Check sheet for the modelled part. Datum: model origin and axes. Units: mm. A direction names the side the tool comes from. Give positions to 0.01 mm unless a question says otherwise; leave off trailing zeros. Loops run counter-clockwise (first coordinate to the right, second up) from the corner with the lowest first, then second, coordinate; pieces in that order, holes last. Notation, with made-up numbers: (70, -7.5) - (101, -7.5) arc R21 cw to (101, -2.5) - close; hole circle Ø3 at (-20, 8.25). An arc over 180 degrees is marked (long way). Use one line per item in the form item = value.
from build123d import *

# Parameters (mm, degrees)
F0_W     = 698.5
F0_H     = 787.4
F1_DEPTH = 6.35
F2_W     = 660.4
F2_H     = 19.05
F3_DEPTH = 228.6
F4_W     = 152.4
F4_H     = 76.2
F5_DEPTH = 25.4


with BuildPart() as f1:
    # F0 (on Front) → F1 (new body)
    with BuildSketch(Plane.XZ):
        with Locations((349.25, 393.7)):
            Rectangle(F0_W, F0_H)
    extrude(amount=F1_DEPTH)

    # F2 (on face) → F3 (join)
    with BuildSketch(Plane.XZ.offset(6.35)):
        Polygon((19.05, 787.4), (0, 787.4), (0, 0), (19.05, 0), (19.05, 19.05), (19.05, 228.6), (19.05, 247.65), (19.05, 457.2), (19.05, 476.25), (19.05, 685.8), (19.05, 704.85), align=None)
        Polygon((698.5, 787.4), (679.45, 787.4), (679.45, 704.85), (679.45, 685.8), (679.45, 476.25), (679.45, 457.2), (679.45, 247.65), (679.45, 228.6), (679.45, 19.05), (679.45, 0), (698.5, 0), align=None)
        with Locations((349.25, 695.325)):
            Rectangle(F2_W, F2_H)
        with Locations((349.25, 466.725)):
            Rectangle(F2_W, F2_H)
        with Locations((349.25, 238.125)):
            Rectangle(F2_W, F2_H)
        with Locations((349.25, 9.525)):
            Rectangle(F2_W, F2_H)
    extrude(amount=F3_DEPTH)

    # F4 (on face) → F5 (cut)
    with BuildSketch(Plane.XZ.offset(6.35)):
        with Locations((349.25, 768.35)):
            Rectangle(F4_W, F4_H)
        with Locations((349.25, 82.55)):
            Rectangle(F4_W, F4_H)
    extrude(amount=-F5_DEPTH, mode=Mode.SUBTRACT)


solid = f1.part
Item 1: Thickness scan on L1, parallel to Z at x = 178, y = -180.5; L2, parallel to X at y = -113.5, z = 705; L3, parallel to Y at x = 124, z = 558.5. Record the ranges inside material, lowest first.
Answer block:
L1 = 0 to 19.05, 228.6 to 247.65, 457.2 to 476.25, 685.8 to 704.85
L2 = 0 to 19.05, 679.45 to 698.5
L3 = -6.35 to 0
Item 2: Section check C-C on y = -61.5. Record the boundary of the cut face in (x, z), then the cut area to 3 significant figures.
Answer block:
outline = (0, 0) - (698.5, 0) - (698.5, 787.4) - (679.45, 787.4) - (679.45, 704.85) - (19.05, 704.85) - (19.05, 787.4) - (0, 787.4) - close; hole (19.05, 19.05) - (679.45, 19.05) - (679.45, 228.6) - (19.05, 228.6) - close; hole (19.05, 247.65) - (679.45, 247.65) - (679.45, 457.2) - (19.05, 457.2) - close; hole (19.05, 476.25) - (679.45, 476.25) - (679.45, 685.8) - (19.05, 685.8) - close
area = 80,300 mm2
Item 3: Section check D-D on x = 477.5. Record the boundary of the cut face in (y, z).
Answer block:
outline = (-234.95, 0) - (0, 0) - (0, 787.4) - (-6.35, 787.4) - (-6.35, 704.85) - (-234.95, 704.85) - (-234.95, 685.8) - (-6.35, 685.8) - (-6.35, 476.25) - (-234.95, 476.25) - (-234.95, 457.2) - (-6.35, 457.2) - (-6.35, 247.65) - (-234.95, 247.65) - (-234.95, 228.6) - (-6.35, 228.6) - (-6.35, 19.05) - (-234.95, 19.05) - close
Item 4: Mould release check, pull along Z, two halves, no side actions. Record for faces 1 (the face through (344, -116, 0)), 2 (the face through (345, -6.35, 728)), 3 (the face through (345, -6.35, 582)): released by +Z, released by -Z, zero draft, split by the parting line, or undercut.
Answer block:
face_1 = released by -Z
face_2 = zero draft
face_3 = undercut
Item 5: Access from +Z, -Z, +X, -X, +Y, -Y to the whole of each face (thin tool, end or side, straight path). Record for faces 4 (the face through (345, -119, 247.65)), 5 (the face through (348, -234.95, 687)).
Answer block:
face_4 = -Y
face_5 = +Z, -Z, +X, -X, -Y
Item 6: Section check B-B on x = 286. Record the boundary of the cut face in (y, z), then the cut area to 3 significant figures.
Answer block:
outline = (-234.95, 0) - (0, 0) - (0, 44.45) - (-6.35, 44.45) - (-6.35, 19.05) - (-234.95, 19.05) - close; (-234.95, 228.6) - (-6.35, 228.6) - (-6.35, 120.65) - (0, 120.65) - (0, 730.25) - (-6.35, 730.25) - (-6.35, 704.85) - (-234.95, 704.85) - (-234.95, 685.8) - (-6.35, 685.8) - (-6.35, 476.25) - (-234.95, 476.25) - (-234.95, 457.2) - (-6.35, 457.2) - (-6.35, 247.65) - (-234.95, 247.65) - close
area = 21,600 mm2
Item 7: Section check A-A on z = 72.5. Record the boundary of the cut face in (x, y), then the cut area to 3 significant figures.
Answer block:
outline = (0, -234.95) - (19.05, -234.95) - (19.05, -6.35) - (273.05, -6.35) - (273.05, 0) - (0, 0) - close; (425.45, -6.35) - (679.45, -6.35) - (679.45, -234.95) - (698.5, -234.95) - (698.5, 0) - (425.45, 0) - close
area = 12,200 mm2
Item 8: Gauge pin test, flat ends, axial feed: P1, Ø1.9, axis at x = 359.5, y = -2, coming from the +Z side; P2, Ø6, axis at x = 114.5, y = -182, coming from the +Z side; P3, Ø25, axis at x = 192, z = 766.5, coming from the -Y side. Record the tip position at first contact, or that the pin passes through.
Answer block:
P1 = 730.25
P2 = 704.85
P3 = -6.35
